Autodesk Inventor part; units mm, degrees
ref_plane "YZ Plane" through (0, 0, 0) normal (1, 0, 0) x (0, 1, 0)
ref_plane "XZ Plane" through (0, 0, 0) normal (0, 1, 0) x (-1, 0, 0)
ref_plane "XY Plane" through (0, 0, 0) normal (0, 0, 1) x (1, 0, 0)
sketch "Sketch1" plane through (0, 0, 0) normal (0, 1, 0) x (-1, 0, 0)
  line L0 (0, 0) -> (-304.8, 0)
  line L1 (-304.8, 0) -> (-304.8, -304.8)
  line L2 (-304.8, -304.8) -> (0, -304.8)
  line L3 (0, -304.8) -> (0, 0)
  dimension "d0" = 304.8
  dimension "d1" = 304.8
extrude "Extrusion1" add sketch "Sketch1" along normal blind 9
sketch "Sketch3" plane through (0, 9, 0) normal (0, 1, 0) x (1, 0, 0)
  line L0 (197.0873, 95) -> (302.0873, 95)
  line L1 (302.0873, 18.175) -> (197.0873, 18.175)
  line L2 (153.4243, 27.425) -> (153.4243, 72.575)
  line L3 (304.8, 0) -> (304.8, 304.8)
  line L4 (304.8, 100) -> (146.4243, 100)
  line L5 (146.4243, 100) -> (146.4243, 0)
  line L6 (146.4243, 0) -> (304.8, 0)
  line L7 (304.8, 0) -> (304.8, 100)
  point P0 (0, 0)
  dimension "d8" = 5
  dimension "d9" = 7
extrude "Extrusion3" cut sketch "Sketch3" against normal blind 10
sketch "Sketch4" plane through (0, 9, 0) normal (0, 1, 0) x (1, 0, 0)
  circle A0 centre (15, 17) radius 3.1
  circle A1 centre (15, 288.8) radius 3.1
  circle A2 centre (289.8, 287.7367) radius 3.1
  circle A3 centre (289.8, 112.4) radius 3.1
  point P0 (0, 0)
extrude "Extrusion4" cut sketch "Sketch4" against normal through all
sketch "Sketch2" plane through (0, 9, 0) normal (0, 1, 0) x (1, 0, 0)
  line L0 (304.8, 304.8) -> (0, 304.8)
  line L1 (304.8, 304.8) -> (144.8, 304.8)
  line L2 (144.8, 304.8) -> (144.8, 209.8)
  line L3 (144.8, 209.8) -> (304.8, 209.8)
  line L4 (304.8, 209.8) -> (304.8, 304.8)
  point P0 (0, 0)
  dimension "d4" = 95
  dimension "d5" = 160
properties part number "acrylic_cover"
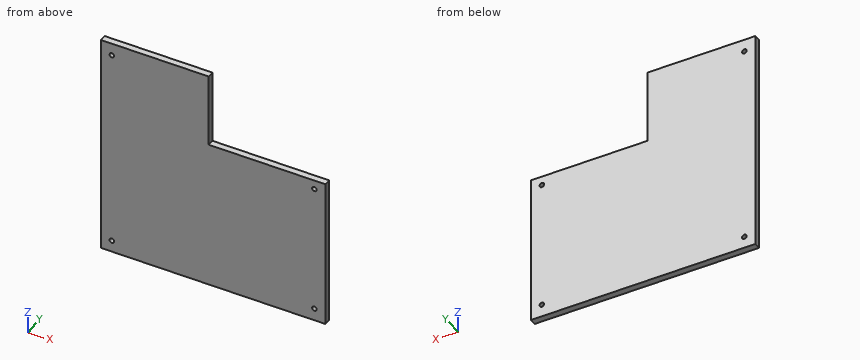
The listing builds one solid part. Answer for the finished solid, in the listing's coordinates (mm). Give positions to 0.01 mm unless a question says otherwise; leave off trailing zeros. Write each loop counter-clockwise with the first axis right and the second up, starting at its lowest first coordinate (ties: lowest second). Pieces come first, ordered by that corner, then holes.
Item 1: A flat-ended cylindrical pin translates along its axis: P1, Ø3, axis at x = 199, y = 4, coming from the +Z side. Find the tip coordinate at first contact, or state that the pin passes through.
Item 2: Section C-C, the plane x = 170.5 is taken. Write down the section's boundary in (y, z).
Item 3: Find the intervals of material crossed by line 1 along Z through (x, y) = (289.8, 5.25); line 2 along X through (y, z) = (7.25, -112.4); line 3 along Z through (x, y) = (15, 2), in increasing order.
Item 4: Section B-B, the plane z = -63 is taken. Write down the section's boundary in (x, y), plus the area to 3 significant figures.
Item 5: Section A-A, the plane y = 4.25 is taken. Write down the section's boundary in (x, z).
Completed:
1. P1: stops at z = -100
2. outline: (0, -304.8) - (9, -304.8) - (9, -100) - (0, -100) - close
3. line 1: z = -304.8 to -290.84, -284.64 to -115.5, -109.3 to -100
3. line 2: x = 0 to 286.7, 292.9 to 304.8
3. line 3: z = -304.8 to -291.9, -285.7 to -20.1, -13.9 to 0
4. outline: (0, 0) - (146.42, 0) - (146.42, 9) - (0, 9) - close
4. area: 1,320 mm2
5. outline: (0, -304.8) - (304.8, -304.8) - (304.8, -100) - (146.42, -100) - (146.42, 0) - (0, 0) - close; hole circle Ø6.2 at (15, -288.8); hole circle Ø6.2 at (15, -17); hole circle Ø6.2 at (289.8, -287.74); hole circle Ø6.2 at (289.8, -112.4)
